```python
from build123d import *

# Parameters (mm, degrees)
SKETCH1_R           = 1.375
BOSS_EXTRUDE1_DEPTH = 6
BOSS_EXTRUDE2_START = 5.865
SKETCH9_W           = 3.5
SKETCH9_H           = 3
BOSS_EXTRUDE2_DEPTH = 7.26
BOSS_EXTRUDE3_START = -26.75
SKETCH10_W          = 3
SKETCH10_H          = 3
BOSS_EXTRUDE3_DEPTH = 23.25
SKETCH11_W          = 3
SKETCH11_H          = 3
BOSS_EXTRUDE4_DEPTH = 5
FILLET1_R           = 2.5
FILLET2_R           = 1


with BuildPart() as part:
    # Sketch1 → Boss-Extrude1 (new body)
    with BuildSketch(Plane(origin=(0, 0, 0), x_dir=(0, 1, 0), z_dir=(0, 0, 1))):
        with BuildLine():
            Line((0, 2.875), (7, 2.875))
            Line((7, 2.875), (7, -2.875))
            Line((7, -2.875), (0, -2.875))
            ThreePointArc((0, -2.875), (-2.875, 0), (0, 2.875))
        make_face()
        with Locations(Location((0, 0, 0), (0, 0, 270))):
            Circle(SKETCH1_R, mode=Mode.SUBTRACT)
    extrude(amount=BOSS_EXTRUDE1_DEPTH)

    # Sketch2 → Loft1 section 0
    with BuildSketch(Plane(origin=(0, 0, 0), x_dir=(1, 0, 0), z_dir=(0, 0, -1))):
        with BuildLine():
            Line((2.875, -7), (-0.875, -7))
            Line((-0.875, -7), (-0.875, -3.5))
            Line((-0.875, -3.5), (2.875, -3.5))
            Line((2.875, -3.5), (2.875, -7))
        make_face()
    # Sketch8 → Loft1 section 1
    with BuildSketch(Plane(origin=(0, 0, -37.5), x_dir=(-1, 0, 0), z_dir=(0, 0, -1))):
        with BuildLine():
            Line((-6.125, 3.5), (-6.125, 7))
            Line((-6.125, 7), (-2.375, 7))
            Line((-2.375, 7), (-2.375, 3.5))
            Line((-2.375, 3.5), (-6.125, 3.5))
        make_face()
    loft()

    # Sketch9 → Boss-Extrude2 (add)
    with BuildSketch(Plane.YZ.offset(BOSS_EXTRUDE2_START)):
        with Locations((5.25, -36)):
            Rectangle(SKETCH9_W, SKETCH9_H)
    extrude(amount=BOSS_EXTRUDE2_DEPTH)

    # Sketch10 → Boss-Extrude3 (add)
    with BuildSketch(Plane(origin=(0, 7, 0), x_dir=(-1, 0, 0), z_dir=(0, 1, 0)).offset(BOSS_EXTRUDE3_START)):
        with Locations((-11.625, -36)):
            Rectangle(SKETCH10_W, SKETCH10_H)
    extrude(amount=BOSS_EXTRUDE3_DEPTH)

    # Sketch11 → Boss-Extrude4 (add)
    with BuildSketch(Plane.XY.offset(-34.5)):
        with Locations((11.625, -18.25)):
            Rectangle(SKETCH11_W, SKETCH11_H)
    extrude(amount=BOSS_EXTRUDE4_DEPTH)

    # Fillet1
    fillet1_edges = [part.edges().sort_by_distance(p)[0] for p in [
        (2.375, 5.25, -37.5),
        (13.125, 7, -36),
        (11.625, -19.75, -37.5),
        (10.125, 3.5, -36),
    ]]
    fillet(fillet1_edges, radius=FILLET1_R)

    # Fillet2
    fillet2_edges = [part.edges().sort_by_distance(p)[0] for p in [
        (0, 7, 6),
        (1, 3.5, 0),
        (5.865, 5.25, -34.5),
        (11.625, -16.75, -34.5),
        (11.625, -19.75, -29.5),
        (13.125, -18.25, -29.5),
        (11.625, -16.75, -29.5),
        (10.125, -18.25, -29.5),
    ]]
    fillet(fillet2_edges, radius=FILLET2_R)


solid = part.part
```
The listing builds one solid part. Answer for the finished solid, in the listing's coordinates (mm). A direction names the side the tool comes from. Give positions to 0.01 mm unless a question says otherwise; leave off trailing zeros. Loops run counter-clockwise (first coordinate to the right, second up) from the corner with the lowest first, then second, coordinate; pieces in that order, holes last. Notation, with made-up numbers: (35.5, 40.5) - (40.5, 40.5) arc R14 cw to (40.5, 51.5) - close; hole circle Ø9 at (10.5, 80.5). An arc over 180 degrees is marked (long way). Answer as CSV lines item,"result". Start each with the question number.
Item 1: Each of these flat-tipped pins is pushed along its axis until it touches: pin 1 (3.5 mm diameter, centred on y = -6, z = -33.5, fed in from -X) (3 decimals); pin 2 (4 mm diameter, centred on x = 2, z = -16, fed in from -Y); pin 3 (2 mm diameter, centred on x = 8, y = -10.5, fed in from -Z); pin 4 (1.1 mm diameter, centred on x = 12, y = -18, fed in from +Z). Where does it stop, or does it pass through?
Item 2: A cutting plane is placed at B-B on x = 0. Determine the outline of the cut face in (y, z) (3 decimals).
Item 3: A cutting plane is placed at D-D on z = -2. Determine the outline of the cut face in (x, y).
Item 4: The mould has two halves that part along X. Classify faces 5 (the face through (-2.875, 3, 3)), 6 (the face through (12.41, 6.25, -35.98)), 7 (the face through (-1, 2, 0)), 8 (the face through (-0.3, -1.34, 2.96)): +X half, -X half, draft (parallel to the pull), parting line (faces both ways), or undercut.
Item 5: A cutting plane is placed at C-C on y = -14.25. Determine the outline of the cut face in (x, z) (3 decimals).
Item 6: A cutting plane is placed at A-A on y = 0.5. Determine the outline of the cut face in (x, z) (3 decimals).
Item 7: Find the intervals of material crossed by line 1 (Y direction, x = 0, z = 3.3) (3 decimals); line 2 (Y direction, x = 5.5, z = -33.5); line 3 (Z direction, x = 11.75, y = -10), in increasing order. Write a range as from..to.
Item 8: For faces 1 (the face through (11.646, -19.563, -29.917)), 2 (the face through (11, -2, -34.5)), 3 (the face through (10.125, -10, -36)), 4 (the face through (12, -16.75, -32)), determine the directions among +Z, -Z, +X, -X, +Y, -Y from which every point of the face is accessible in a straight line to the end or side of a thin tool.
Found:
1,pin 1,"stops at x = 10.125"
1,pin 2,"stops at y = 3.5"
1,pin 3,"passes through"
1,pin 4,"stops at z = -29.5"
2,outline,"(-2.875, 0) - (-1.375, 0) - (-1.375, 6) - (-2.875, 6) - close; (1.375, 0) - (2.5, 0) arc R1 cw to (3.5, -1) - (3.5, -10.096) - (7, -10.096) - (7, 5) arc R1 ccw to (6, 6) - (1.375, 6) - close"
3,outline,"(-0.7, 3.5) - (3.05, 3.5) - (3.05, 7) - (-0.7, 7) - close"
4,face 5,"-X half"
4,face 6,"+X half"
4,face 7,"draft"
4,face 8,"undercut"
5,outline,"(10.125, -37.5) - (13.125, -37.5) - (13.125, -34.5) - (10.125, -34.5) - close"
6,outline,"(-2.875, 0) - (-1.281, 0) - (-1.281, 6) - (-2.875, 6) - close; (1.281, 0) - (2.875, 0) - (2.875, 6) - (1.281, 6) - close; (10.125, -37.5) - (13.125, -37.5) - (13.125, -34.5) - (10.125, -34.5) - close"
7,line 1,"y = -2.875..-1.375, 1.375..7"
7,line 2,"y = 3.5..7"
7,line 3,"z = -37.5..-34.5"
8,face 1,"+Z, +X, -X, -Y"
8,face 2,"+Z, +X, +Y"
8,face 3,"+Z, -Z, -X, -Y"
8,face 4,"+Z, +X, -X, +Y"
